The model under review builds one solid part; all positions refer to its coordinate system, in mm. A direction names the side the tool comes from. Round coordinates to 2 decimals unless told otherwise and drop trailing zeros. Loops run counter-clockwise (first coordinate to the right, second up) from the corner with the lowest first, then second, coordinate; pieces in that order, holes last. Notation, with made-up numbers: (-2.5, 67) -> (56.5, 67) arc R29 cw to (56.5, 98) -> close; hole circle Ø7 at (15.5, 85.5). An arc over 180 degrees is marked (long way). Use a Markdown table: item, result. Add a question column.
1) Consider section C-C on x = -29.5. Give the boundary of the cut face in (y, z), plus the area to 3 significant figures.
2) For faces 1 (the flat face through (15, 15, 25)), 2 (the flat face through (42.3, 47, 12)), 3 (the flat face through (-14, -4, 12)), 4 (the flat face through (42.3, -18, 12)), 5 (the flat face through (0, 34, 12)), list the 3-axis set-ups (+Z, -Z, +X, -X, +Y, -Y) from which the entire face can be reached by the end or side of a thin tool; tool diameter is ignored.
3) Consider section B-B on z = 7.75. Give the boundary of the cut face in (x, y), plus the area to 3 significant figures.
4) Consider section D-D on x = 10. Give the boundary of the cut face in (y, z), plus the area to 3 significant figures.
5) Mouldability with a two-part tool opening along X and no side actions: class faces 6 (the flat face through (56.3, 14, 12)), 7 (the flat face through (0, -5, 12)), 8 (the flat face through (21.45, 39.91, 12.32)) as released by +X, released by -X, zero draft, split by the parting line, or undercut.
6) Consider section A-A on y = -3. Give the boundary of the cut face in (x, z), plus the area to 3 significant figures.
7) Insertion check: pin 1 (8 mm diameter, centred on x = 29, z = 16, fed in from +Y); pin 2 (4 mm diameter, centred on x = -3, z = 22, fed in from +Y); pin 3 (5 mm diameter, centred on x = 34.5, z = 20, fed in from +Y). Each pin has a flat end and moves straight along its axis. Give the tip position at first contact, or say it passes through.
8) Wall thickness on probe 1 along X at (y, z) = (45, 1.75); probe 2 along Y at (x, z) = (-7.5, 7.75); probe 3 along X at (y, z) = (-7.5, 17.25): over which ranges is each line inside the solid? List them lowest first.
from build123d import *

# Parameters (mm, degrees)
F1_DEPTH = 25


with BuildPart() as f1:
    # F0 (on Top) → F1 (new body)
    with BuildSketch(Plane.XY):
        with BuildLine():
            Line((56.300399, -20.339935), (56.300399, 49.660065))
            ThreePointArc((56.300399, 49.660065), (55.421719, 51.781386), (53.300399, 52.660065))
            Line((53.300399, 52.660065), (43.800399, 52.660065))
            ThreePointArc((43.800399, 52.660065), (42.739739, 52.220726), (42.300399, 51.160065))
            Line((42.300399, 51.160065), (42.300399, 42.660065))
            Line((42.300399, 42.660065), (0, 37.081991))
            Line((0, 37.081991), (0, 30.660065))
            Line((0, 30.660065), (-14, 30.660065))
            Line((-14, 30.660065), (-14, 35.235837))
            Line((-14, 35.235837), (-47.395706, 30.832008))
            ThreePointArc((-47.395706, 30.832008), (-48.327466, 30.333781), (-48.699601, 29.344882))
            Line((-48.699601, 29.344882), (-48.699601, 14.660065))
            Line((-48.699601, 14.660065), (-48.699601, -0.024751))
            ThreePointArc((-48.699601, -0.024751), (-48.327466, -1.01365), (-47.395706, -1.511877))
            Line((-47.395706, -1.511877), (-14, -5.915706))
            Line((-14, -5.915706), (-14, -1.339935))
            Line((-14, -1.339935), (0, -1.339935))
            Line((0, -1.339935), (0, -7.76186))
            Line((0, -7.76186), (42.300399, -13.339935))
            Line((42.300399, -13.339935), (42.300399, -21.839935))
            ThreePointArc((42.300399, -21.839935), (42.739739, -22.900595), (43.800399, -23.339935))
            Line((43.800399, -23.339935), (53.300399, -23.339935))
            ThreePointArc((53.300399, -23.339935), (55.421719, -22.461255), (56.300399, -20.339935))
        make_face()
    extrude(amount=F1_DEPTH)


solid = f1.part
Result set:
| question | item | result |
|---|---|---|
| 1 | outline | (-3.87, 0) -> (33.19, 0) -> (33.19, 25) -> (-3.87, 25) -> close |
| 1 | area | 927 mm2 |
| 2 | face 1 | +Z, +X, -X, +Y, -Y |
| 2 | face 2 | +Z, -Z, -X, +Y |
| 2 | face 3 | +Z, -Z, -Y |
| 2 | face 4 | +Z, -Z, -X, -Y |
| 2 | face 5 | +Z, -Z, +Y |
| 3 | outline | (-48.7, -0.02) arc R1.5 ccw to (-47.4, -1.51) -> (-14, -5.92) -> (-14, -1.34) -> (0, -1.34) -> (0, -7.76) -> (42.3, -13.34) -> (42.3, -21.84) arc R1.5 ccw to (43.8, -23.34) -> (53.3, -23.34) arc R3 ccw to (56.3, -20.34) -> (56.3, 49.66) arc R3 ccw to (53.3, 52.66) -> (43.8, 52.66) arc R1.5 ccw to (42.3, 51.16) -> (42.3, 42.66) -> (0, 37.08) -> (0, 30.66) -> (-14, 30.66) -> (-14, 35.24) -> (-47.4, 30.83) arc R1.5 ccw to (-48.7, 29.34) -> close |
| 3 | area | 4,910 mm2 |
| 4 | outline | (-9.08, 0) -> (38.4, 0) -> (38.4, 25) -> (-9.08, 25) -> close |
| 4 | area | 1,190 mm2 |
| 5 | face 6 | released by +X |
| 5 | face 7 | undercut |
| 5 | face 8 | released by -X |
| 6 | outline | (-36.11, 0) -> (-14, 0) -> (-14, 25) -> (-36.11, 25) -> close; (0, 0) -> (56.3, 0) -> (56.3, 25) -> (0, 25) -> close |
| 6 | area | 1,960 mm2 |
| 7 | pin 1 | y = 41.43 |
| 7 | pin 2 | y = 30.66 |
| 7 | pin 3 | y = 41.96 |
| 8 | probe 1 | 42.3 to 56.3 |
| 8 | probe 2 | -1.34 to 30.66 |
| 8 | probe 3 | 0 to 56.3 |
